from build123d import *

# Parameters (mm, degrees)
SKETCH029_W     = 3.5
SKETCH029_H     = 6.5
PAD023_DEPTH    = 0.9
SKETCH030_W     = 7.5
SKETCH030_H     = 2.5
PAD024_DEPTH    = 1.5
PAD025_DEPTH    = 2.7
SKETCH032_W     = 1.5
SKETCH032_H     = 1.2
POCKET002_DEPTH = 2.5
CHAMFER004_SIZE = 1


with BuildPart() as part:
    # Sketch029 → Pad023 (new body, symmetric)
    with BuildSketch(Plane.XZ):
        with Locations((0, 3.25)):
            Rectangle(SKETCH029_W, SKETCH029_H)
    extrude(amount=PAD023_DEPTH, both=True)

    # Sketch030 (on Face6 of Pad023) → Pad024 (join)
    with BuildSketch(Plane.XZ.offset(0.9)):
        with Locations((0, 6.25)):
            Rectangle(SKETCH030_W, SKETCH030_H)
    extrude(amount=PAD024_DEPTH)

    # Sketch033 (on DatumPlane) → Pad025 (join)
    with BuildSketch(Plane(origin=(0, 0.9, 0), x_dir=(-1, 0, 0), z_dir=(0, 1, 0))):
        Polygon((-1.75, 7.5), (1.75, 7.5), (2.75, 6.5), (2.75, 1.6), (1.75, 0.6), (-1.75, 0.6), (-2.75, 1.6), (-2.75, 6.5), align=None)
    extrude(amount=PAD025_DEPTH)

    # Sketch032 → Pocket002 (cut)
    with BuildSketch(Plane.XZ.offset(0.9)):
        with Locations((0, 3.5)):
            Rectangle(SKETCH032_W, SKETCH032_H)
    extrude(amount=-POCKET002_DEPTH, mode=Mode.SUBTRACT)

    # Chamfer004
    chamfer004_edges = [part.edges().sort_by_distance(p)[0] for p in [
        (2.75, 3.6, 4.05),
        (2.25, 3.6, 7),
        (0, 3.6, 7.5),
        (-2.25, 3.6, 7),
        (-2.75, 3.6, 4.05),
        (-2.25, 3.6, 1.1),
        (0, 3.6, 0.6),
        (2.25, 3.6, 1.1),
    ]]
    chamfer(chamfer004_edges, length=CHAMFER004_SIZE)


with BuildPart() as part_1:
    # Body013 placement: moved
    add(part.part.moved(Location((123.25, 0, 0))))


solid = part_1.part
Verification items for the finished model (mm, model axes). A direction names the side the tool comes from. Coordinates: 2 decimals unless noted, no trailing zeros. Order: outer loops, then holes, each group sorted by start corner. A loop starts at its lowest first (then second) coordinate and runs counter-clockwise, first axis right, second up. Notation, with made-up numbers: M 62,51.5 L 93,51.5 A22 cw 93,59.5 Z; hole C 22.5,-39 d10. An arc over 180 degrees is marked long. One line per item, written item: value. Start each with the question number.
Item 1: Thickness scan on probe 1 along Z at (x, y) = (123.5, -0.5); probe 2 along X at (y, z) = (0.25, 3.25); probe 3 along X at (y, z) = (0.5, 1.25). Record the ranges inside material, lowest first.
Item 2: Depth check by flat-ended pin: P1, Ø1, axis at y = -0.5, z = 3.5, coming from the -X side; P2, Ø0.5, axis at y = 2, z = 4, coming from the +X side; P3, Ø1.4, axis at y = 0.5, z = 3, coming from the -X side. Enter the tip coordinate at first touch or a pass-through.
Item 3: Sectioned sample at A-A on z = 5.5. Record the cut outline in (x, y), then the cut area to 3 significant figures.
Item 4: Sectioned sample at B-B on y = -0.75. Record the cut outline in (x, z).
Item 5: Access from +Z, -Z, +X, -X, +Y, -Y to the whole of each face (thin tool, end or side, straight path). Record for faces 1 (the flat face through (124, 0.3, 3.5)), 2 (the flat face through (123, -0.9, 7)), 3 (the flat face through (126, 2, 4)).
Item 6: Sectioned sample at C-C on y = 2.25. Record the cut outline in (x, z), then the cut area to 4 significant figures.
Item 7: Mould release check, pull along Z, two halves, no side actions. Record for faces 4 (the flat face through (125.5, 1.7, 1.1)), 5 (the flat face through (123, 3.6, 4)), 6 (the flat face through (123.2, 1.6, 3.5)): pulls with the +Z half, pulls with the -Z half, needs draft (parallel to the pull), parting line crosses it, or undercut.
Item 8: Sectioned sample at D-D on x = 121.75. Record the cut outline in (y, z), then the cut area to 3 significant figures.
Calculated:
1. probe 1: 0 to 2.9, 4.1 to 6.5
1. probe 2: 121.5 to 122.5, 124 to 125
1. probe 3: 121.5 to 125
2. P1: x = 121.5
2. P2: x = 126
2. P3: x = 120.5
3. outline: M 119.5,-2.4 L 127,-2.4 L 127,-0.9 L 125,-0.9 L 125,0.9 L 126,0.9 L 126,2.6 L 125,3.6 L 121.5,3.6 L 120.5,2.6 L 120.5,0.9 L 121.5,0.9 L 121.5,-0.9 L 119.5,-0.9 Z
3. area: 31.4 mm^2
4. outline: M 121.5,0 L 125,0 L 125,6.5 L 121.5,6.5 Z; hole M 122.5,2.9 L 124,2.9 L 124,4.1 L 122.5,4.1 Z
5. face 1: -Y
5. face 2: +Z
5. face 3: +Z, -Z, +X, +Y
6. outline: M 120.5,1.6 L 121.5,0.6 L 125,0.6 L 126,1.6 L 126,6.5 L 125,7.5 L 121.5,7.5 L 120.5,6.5 Z
6. area: 35.95 mm^2
7. face 4: pulls with the -Z half
7. face 5: needs draft
7. face 6: undercut
8. outline: M -2.4,5 L -0.9,5 L -0.9,0 L 0.9,0 L 0.9,0.6 L 2.6,0.6 L 3.2,1.2 L 3.6,1.76 L 3.6,6.34 L 3.2,6.9 L 2.6,7.5 L 0.9,7.5 L 0.9,6.5 L -0.9,6.5 L -0.9,7.5 L -2.4,7.5 Z
8. area: 33.0 mm^2
